from build123d import *

# Parameters (mm, degrees)
CHAMFER_1_SIZE = 0.5


with BuildPart() as part:
    # Эскиз1 → Повернуть1 (revolve)
    with BuildSketch(Plane.XY, mode=Mode.PRIVATE) as revolve_1_sk:
        Polygon((50.9, 4), (52, 4), (52, 0), (0, 0), (-5, 0), (-5, 8), (0, 8), (0, 5), (29, 5), (29, 4), (50, 4), (50, 3.8), (50.9, 3.8), align=None)
    revolve(revolve_1_sk.sketch.rotate(Axis((0, 0, 0), (1, 0, 0)), 90), axis=Axis((0, 0, 0), (1, 0, 0)))

    # Фаска1
    chamfer_1_edges = [part.edges().sort_by_distance(p)[0] for p in [
        (52, 0, -4),
    ]]
    chamfer(chamfer_1_edges, length=CHAMFER_1_SIZE)


solid = part.part
Input: part model. Units: mm. Frame: model coordinates. A direction names the side the tool comes from. Coordinates: 2 decimals unless noted, no trailing zeros. Order: outer loops, then holes, each group sorted by start corner. A loop starts at its lowest first (then second) coordinate and runs counter-clockwise, first axis right, second up. Notation, with made-up numbers: M 56,-23 L 68,-23 A20 ccw 68,-8 Z; hole C -11.75,-12 d4. An arc over 180 degrees is marked long. One line per question, with ' | ' between items.
Item 1: Draft query along X for faces 1 (the flat face through (0, 5.2, -0.1)), 2 (the cylindrical face through (50.456, -1.141, 3.625)), 3 (the cylindrical face through (15, 0, -5)). Return one class per face: released by +X, released by -X, zero draft, split by the parting line, or undercut.
Geometry results:
face 1: released by +X | face 2: undercut | face 3: zero draft
Item 2: Pin query (flat end, axial travel): pin 1 (3 mm diameter, centred on x = 4.5, z = 1.5, fed in from -Y); pin 2 (8 mm diameter, centred on x = 5.5, y = 1, fed in from -Z); pin 3 (1.5 mm diameter, centred on x = 39.5, z = 0.5, fed in from +Y). Return the tip coordinate at first contact, or that it passes through.
Geometry results:
pin 1: stops at y = -5 | pin 2: stops at z = -5 | pin 3: stops at y = 4
Item 3: Ray query, line 1 along X through (y, z) = (-2.5, 4.75); line 2 along Z through (x, y) = (0.5, -0.25); line 3 along Y through (x, z) = (23.5, 0). Return the intervals inside material, ascending.
Geometry results:
line 1: x = -5 to 0 | line 2: z = -4.99 to 4.99 | line 3: y = -5 to 5
Item 4: Section C-C (x = 44.5). Output: boundary loops of the cut face in (y, z).
Geometry results:
outline: C 0,0 d8
Item 5: Section D-D (y = 4.5). Output: boundary loops of the cut face in (x, z).
Geometry results:
outline: M -5,-6.61 L 0,-6.61 L 0,-2.18 L 29,-2.18 L 29,2.18 L 0,2.18 L 0,6.61 L -5,6.61 Z
Item 6: Reachability of faces 4 (the cylindrical face through (39.647, 3.905, -0.867)), 5 (the flat face through (-5, 0, 0)) from +Z, -Z, +X, -X, +Y, -Y: full face, straight path, thin tool, end or side. Return the list, or none.
Geometry results:
face 4: +X | face 5: +Z, -Z, -X, +Y, -Y
Item 7: Section A-A (z = 0). Output: boundary loops of the cut face in (x, y).
Geometry results:
outline: M -5,-8 L 0,-8 L 0,-5 L 29,-5 L 29,-4 L 50,-4 L 50,-3.8 L 50.9,-3.8 L 50.9,-4 L 51.5,-4 L 52,-3.5 L 52,3.5 L 51.5,4 L 50.9,4 L 50.9,3.8 L 50,3.8 L 50,4 L 29,4 L 29,5 L 0,5 L 0,8 L -5,8 Z
